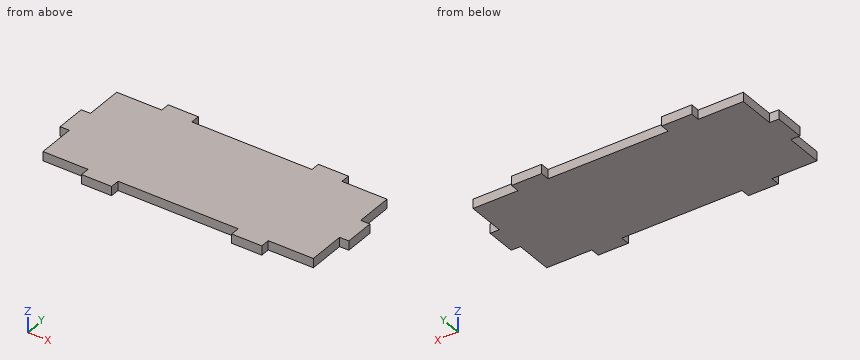
```python
from build123d import *

# Parameters (mm, degrees)
F2_DEPTH = 6.14


# Not quite as in the source:
# - a feature names something its author has since deleted; it is built from what else it names


with BuildPart() as f2:
    # F1 (on Top) → F2 (new body)
    with BuildSketch(Plane.XY):
        Polygon((90, 10), (90, 35), (60, 35), (60, 41.14), (40, 41.14), (40, 35), (-40, 35), (-40, 41.14), (-60, 41.14), (-60, 35), (-90, 35), (-90, 10), (-96.14, 10), (-96.14, -10), (-90, -10), (-90, -35), (-60, -35), (-60, -41.14), (-40, -41.14), (-40, -35), (40, -35), (40, -41.14), (60, -41.14), (60, -35), (90, -35), (90, -10), (96.14, -10), (96.14, 10), align=None)
    extrude(amount=F2_DEPTH)


solid = f2.part
```
Geometry: final body of the model. Coordinates: model frame, mm. Give positions to 0.01 mm unless a question says otherwise; leave off trailing zeros. Loops run counter-clockwise (first coordinate to the right, second up) from the corner with the lowest first, then second, coordinate; pieces in that order, holes last. Notation, with made-up numbers: (11.25, 32) -> (66.25, 32) arc R18 ccw to (66.25, 65) -> close; hole circle Ø4 at (70.25, 31.25). An arc over 180 degrees is marked (long way). Return JSON: item names as keys, results as strings.
Item 1: Pin query (flat end, axial travel): P1, Ø1.8, axis at y = -18, z = 2.5, coming from the -X side; P2, Ø3, axis at x = -68.5, z = 4, coming from the +Y side; P3, Ø1.8, axis at y = -37, z = 4, coming from the -X side. Return the tip coordinate at first contact, or that it passes through.
Filled in:
{"P1": "x = -90", "P2": "y = 35", "P3": "x = -60"}
Item 2: Line query: line 1 (X direction, y = 36.5, z = 3.25); line 2 (Y direction, x = -81, z = 4); line 3 (X direction, y = 12.5, z = 3). Output: solid intervals per line, ascending.
Filled in:
{"line 1": "-60 to -40, 40 to 60", "line 2": "-35 to 35", "line 3": "-90 to 90"}
Item 3: Section A-A, the plane z = 1.5. Output: boundary loops of the cut face in (x, y).
Filled in:
{"outline": "(-96.14, -10) -> (-90, -10) -> (-90, -35) -> (-60, -35) -> (-60, -41.14) -> (-40, -41.14) -> (-40, -35) -> (40, -35) -> (40, -41.14) -> (60, -41.14) -> (60, -35) -> (90, -35) -> (90, -10) -> (96.14, -10) -> (96.14, 10) -> (90, 10) -> (90, 35) -> (60, 35) -> (60, 41.14) -> (40, 41.14) -> (40, 35) -> (-40, 35) -> (-40, 41.14) -> (-60, 41.14) -> (-60, 35) -> (-90, 35) -> (-90, 10) -> (-96.14, 10) -> close"}
Item 4: Section B-B, the plane x = 32. Output: boundary loops of the cut face in (y, z), plus the area to 3 significant figures.
Filled in:
{"outline": "(-35, 0) -> (35, 0) -> (35, 6.14) -> (-35, 6.14) -> close", "area": "430 mm^2"}
Item 5: Section C-C, the plane y = 31.5. Output: boundary loops of the cut face in (x, z).
Filled in:
{"outline": "(-90, 0) -> (90, 0) -> (90, 6.14) -> (-90, 6.14) -> close"}
